Can you work these out from the model? Positions are in its coordinate system, mm. A direction names the side the tool comes from. Coordinates: 2 decimals unless noted, no trailing zeros. Loops run counter-clockwise (first coordinate to the right, second up) from the corner with the lowest first, then second, coordinate; pieces in that order, holes last. Notation, with made-up numbers: (70, 87) -> (99, 87) arc R8 cw to (99, 97) -> close; hole circle Ø2 at (49.25, 46.5). An arc over 180 degrees is marked (long way). Use one line per item in the form item = value. Start each with the question number.
(1) On a 3-axis mill with a long thin cutter (end or side, diameter ignored), from which of +Z, -Z, +X, -X, +Y, -Y can I reach the whole of each face in a straight line? I mean faces 4 (the flat face through (120, -33, -35.941)), 5 (the flat face through (120, -95, 27.559)), 6 (the flat face through (120, -63.5, -42)). Say none if no direction works.
(2) Imagine slicing it at A-A (x = 146). List the corners of the cut face in (y, z) for me.
(3) Thinking about a two-plate mould opening in Y: for faces 1 (the flat face through (57.531, -51, -4)), 2 (the flat face through (44.831, -50, -11)), 3 (the flat face through (120, 0, -10)), which applies, released by +Y, released by -Y, zero draft, split by the parting line, or undercut?
(4) I need wall thicknesses on line 1 (X direction, y = -51.5, z = 5.5); line 2 (X direction, y = -40, z = -45); line 3 (Y direction, x = 60.5, z = -11). Which ranges of each line are inside material? Lowest first, please. Write a range as [from, to].
(5) Imagine slicing it at B-B (y = -47.5). List the corners of the cut face in (x, z) for me.
(6) I'm going to push a flat-ended pin straight in: pin 1 (3 mm diameter, centred on x = 106, y = -23.5, fed in from +Z). Where does the tip first touch, or does it pass through?
(7) Imagine slicing it at D-D (x = 74.5). List the corners of the cut face in (y, z) for me.
(8) Imagine slicing it at C-C (z = 0). List the corners of the cut face in (x, y) for me.
```python
from build123d import *

# Parameters (mm, degrees)
F0_W     = 152.4
F0_H     = 76.2
F1_DEPTH = 101.6
F2_W     = 127
F2_H     = 76.2
F3_DEPTH = 63.5
F4_W     = 76.2
F4_H     = 25.4
F5_DEPTH = 12.7


with BuildPart() as f1:
    # F0 (on Front) → F1 (new body)
    with BuildSketch(Plane.XZ):
        with Locations((121.03101, -10.541003)):
            Rectangle(F0_W, F0_H)
    extrude(amount=F1_DEPTH)

    # F2 (on face) → F3 (cut)
    with BuildSketch(Plane.XY.offset(27.558997)):
        with Locations((121.03101, -50.8)):
            Rectangle(F2_W, F2_H)
    extrude(amount=-F3_DEPTH, mode=Mode.SUBTRACT)

    # F4 (on face) → F5 (cut)
    with BuildSketch(Plane.XY.offset(-35.941003)):
        with Locations((121.03101, -50.8)):
            Rectangle(F4_W, F4_H)
    extrude(amount=-F5_DEPTH, mode=Mode.SUBTRACT)


solid = f1.part
```
Worked out:
q1.face_4 = +Z
q1.face_5 = +Z, +X, -X, +Y, -Y
q1.face_6 = +Z, -Z
q2.outline = (-101.6, -48.64) -> (-63.5, -48.64) -> (-63.5, -35.94) -> (-88.9, -35.94) -> (-88.9, 27.56) -> (-101.6, 27.56) -> close; (-38.1, -48.64) -> (0, -48.64) -> (0, 27.56) -> (-12.7, 27.56) -> (-12.7, -35.94) -> (-38.1, -35.94) -> close
q3.face_1 = undercut
q3.face_2 = zero draft
q3.face_3 = released by +Y
q4.line_1 = [44.83, 57.53], [184.53, 197.23]
q4.line_2 = [44.83, 82.93], [159.13, 197.23]
q4.line_3 = [-101.6, -88.9], [-12.7, 0]
q5.outline = (44.83, -48.64) -> (82.93, -48.64) -> (82.93, -35.94) -> (57.53, -35.94) -> (57.53, 27.56) -> (44.83, 27.56) -> close; (159.13, -48.64) -> (197.23, -48.64) -> (197.23, 27.56) -> (184.53, 27.56) -> (184.53, -35.94) -> (159.13, -35.94) -> close
q6.pin_1 = -35.94
q7.outline = (-101.6, -48.64) -> (0, -48.64) -> (0, 27.56) -> (-12.7, 27.56) -> (-12.7, -35.94) -> (-88.9, -35.94) -> (-88.9, 27.56) -> (-101.6, 27.56) -> close
q8.outline = (44.83, -101.6) -> (197.23, -101.6) -> (197.23, 0) -> (44.83, 0) -> close; hole (57.53, -88.9) -> (184.53, -88.9) -> (184.53, -12.7) -> (57.53, -12.7) -> close
